```python
from build123d import *

# Parameters (mm, degrees)
BASPROSKE_W        = 10
BASPROSKE_H        = 4.4
TOOTHCUT_DEPTH     = 12.777945491
TEETHCUTS_COUNT    = 20
TEETHCUTS_ANGLE    = 342
BORSKE_R           = 1
BORE_DEPTH         = 50.0000508
SKETCH1_W          = 0.51
SKETCH1_H          = 0.51
CUT_EXTRUDE1_DEPTH = 100


with BuildPart() as part:
    # BasProSke → Base-Revolve (revolve)
    with BuildSketch(Plane(origin=(0, 0, 0), x_dir=(1, 0, 0), z_dir=(0, 1, 0)), mode=Mode.PRIVATE) as base_revolve_sk:
        with Locations((5, 2.2)):
            Rectangle(BASPROSKE_W, BASPROSKE_H)
    revolve(base_revolve_sk.sketch.rotate(Axis((-10, 0, 0), (1, 0, 0)), 180), axis=Axis((-10, 0, 0), (1, 0, 0)))

    # TooCutSke → ToothCut (cut, through all)
    with BuildSketch(Plane(origin=(0, 0, 0), x_dir=(0, 0, -1), z_dir=(1, 0, 0))):
        with BuildLine():
            ThreePointArc((0.199592598, 3.493302706), (0, 3.499), (-0.199592598, 3.493302706))
            ThreePointArc((-0.199592598, 3.493302706), (-0.333052166, 3.970347354), (-0.606028648, 4.383707841))
            ThreePointArc((-0.606028648, 4.383707841), (0, 4.4254), (0.606028648, 4.383707841))
            ThreePointArc((0.606028648, 4.383707841), (0.333052166, 3.970347354), (0.199592598, 3.493302706))
        make_face()
    toothcut = extrude(amount=TOOTHCUT_DEPTH, mode=Mode.SUBTRACT)

    # TeethCuts: ToothCut ×20 about axis
    teethcuts_axis = Axis((-10, 0, 0), (1, 0, 0))
    for i in range(1, TEETHCUTS_COUNT):
        add(toothcut.rotate(teethcuts_axis, i * TEETHCUTS_ANGLE / (TEETHCUTS_COUNT - 1)), mode=Mode.SUBTRACT)

    # BorSke → Bore (cut, symmetric)
    with BuildSketch(Plane(origin=(0, 0, 0), x_dir=(0, 0, -1), z_dir=(1, 0, 0))):
        with Locations(Location((0, 0, 0), (0, 0, 180))):
            Circle(BORSKE_R)
    extrude(amount=BORE_DEPTH, both=True, mode=Mode.SUBTRACT)

    # Sketch1 → Cut-Extrude1 (cut)
    with BuildSketch(Plane(origin=(10, 0, 0), x_dir=(0, 0, -1), z_dir=(1, 0, 0))):
        with Locations((0, 1.213665218)):
            Rectangle(SKETCH1_W, SKETCH1_H)
        with Locations((1.213665218, 0)):
            Rectangle(SKETCH1_W, SKETCH1_H)
        with Locations((0, -1.213665218)):
            Rectangle(SKETCH1_W, SKETCH1_H)
        with Locations((-1.213665218, 0)):
            Rectangle(SKETCH1_W, SKETCH1_H)
    extrude(amount=-CUT_EXTRUDE1_DEPTH, mode=Mode.SUBTRACT)


solid = part.part
```
Geometry check sheet. Reference: the model listing, model coordinates, mm. A direction names the side the tool comes from. Coordinates: 2 decimals unless noted, no trailing zeros. Loops run counter-clockwise (first coordinate to the right, second up) from the corner with the lowest first, then second, coordinate; pieces in that order, holes last. Notation, with made-up numbers: (-15.75, 82.25) - (6.25, 82.25) arc R21 cw to (6.25, 114.25) - close; hole circle Ø11 at (46.5, 53). An arc over 180 degrees is marked (long way). One line per item, written item: value. Start each with the question number.
(1) Cross-section at A-A on z = -1.75. Enter the section's corners in (x, y), plus the area to 3 significant figures.
(2) Depth check by flat-ended pin: P1, Ø1.5, axis at x = 3.5, y = 2, coming from the -Z side; P2, Ø0.6, axis at x = 6, z = -1.5, coming from the +Y side; P3, Ø0.6, axis at x = 6, y = 1, coming from the -Z side. Enter the tip coordinate at first touch or a pass-through.
(3) Mould release check, pull along Y, two halves, no side actions. Record for faces 1 (the flat face through (10, 1, -1)), 2 (the cylindrical face through (4.93, -0.913, -3.857)), 3 (the cylindrical face through (4.93, -3.005, -2.584)): released by +Y, released by -Y, zero draft, split by the parting line, or undercut.
(4) Material ranges on line 1 (Z direction, x = 4, y = 3); line 2 (Z direction, x = 4.5, y = -3.75), recorded low to high. Write a range as [from, to].
(5) Tool access check on faces 4 (the cylindrical face through (4.93, 3.005, 2.584)), 5 (the cylindrical face through (4.93, -0.33, -3.96)), 6 (the cylindrical face through (4.93, -2.584, 3.005)), 7 (the cylindrical face through (4.93, -0.91, 3.87)). Record the directions out of +Z, -Z, +X, -X, +Y, -Y that give a thin tool (end or side, any length) a straight path to the whole face; none if there is none.
Results below:
1. outline: (0, -3.86) - (10, -3.86) - (10, 3.86) - (0, 3.86) - close
1. area: 77.2 mm2
2. P1: stops at z = -3.97
2. P2: stops at y = 3.9
2. P3: stops at z = -4.34
3. face 1: zero draft
3. face 2: undercut
3. face 3: released by -Y
4. line 1: z = [-3.17, -2.57], [-1.92, 1.92], [2.57, 3.17]
4. line 2: z = [-2.1, -1.62], [-0.92, -0.25], [0.25, 0.92], [1.62, 2.1]
5. face 4: +X, -X, +Y
5. face 5: -Z, +X, -X
5. face 6: +Z, +X, -X
5. face 7: +X, -X
